Autodesk Inventor part; units mm, degrees
ref_plane "Work Plane1" through (29, 0, 0) normal (0, -1, 0) x (1, 0, 0)
ref_plane "YZ Plane" through (0, 0, 0) normal (1, 0, 0) x (0, 1, 0)
ref_plane "XZ Plane" through (0, 0, 0) normal (0, 1, 0) x (-1, 0, 0)
sketch "Skizze1" plane through (0, 0, 0) normal (0, 0, 1) x (1, 0, 0)
  line L0 (-2, 0) -> (50, 0)
  line L1 (50, 0) -> (50, 4)
  line L2 (50, 4) -> (22, 4)
  line L3 (22, 4) -> (21.2331, 4)
  line L4 (21.2331, 4) -> (0, 4)
  line L5 (0, 4) -> (0, 6.5)
  line L6 (0, 6.5) -> (-8, 6.5)
  line L7 (-8, 6.5) -> (-8, 3.4641)
  line L8 (-8, 3.4641) -> (-4, 3.4641)
  line L9 (-4, 3.4641) -> (-2, 0)
  line L10 (-19.6, 0) -> (61.6, 0)
  line L11 (0, -1.3) -> (0, 7.8)
  line L12 (22, 4) -> (0, 4) construction
  dimension "d1" = 28
  dimension "d2" = 0.7669
  dimension "d3" = 8
  dimension "d4" = 4
  dimension "d5" = 60
  dimension "d6" = 8
  dimension "d7" = 8
  dimension "d8" = 6.9282
  dimension "d9" = 13
  dimension "d26" = 50
revolve "Körper" add sketch "Skizze1" angle 360 about axis through (-2, 0, 0) along (1, 0, 0)
sketch "Skizze2" plane through (-8, 0, 0) normal (-1, 0, 0) x (0, 0, 1)
  circle A0 centre (0, 0) radius 3.4641
  line L0 (0, -9.1) -> (0, 9.1)
  line L1 (-9.1, 0) -> (9.1, 0)
  line L2 (3.4641, 0) -> (1.7321, -3)
  line L3 (1.7321, -3) -> (-1.7321, -3)
  line L4 (-1.7321, -3) -> (-3.4641, 0)
  line L5 (-3.4641, 0) -> (-1.7321, 3)
  line L6 (-1.7321, 3) -> (1.7321, 3)
  line L7 (1.7321, 3) -> (3.4641, 0)
extrude "Loch" add sketch "Skizze2" against normal up to next contours L7 A0 | A0 L2 | L6 L0 A0 | A0 L0 L3 | L0 L6 A0 | A0 L3 L0 | L4 A0 | A0 L5
fillet "Rundung1" radius 0.8 1 edges at (-8, -6.5, 0)
thread "Gewinde"
chamfer "Fase1" distance 0.7668 distance2 0.7668 1 edges at (50, -4, 0) measured on face at (50, -0.3588, -0.308)
ref_plane "Work Plane1" through (29, 0, 0) normal (0, -1, 0) x (1, 0, 0)
fillet "Fillet2" radius 0.4 1 edges at (0, -4, 0)
equation "\"d1\" = GEL"
equation "\"d3\" = KOH"
equation "\"d4\" = INTI"
equation "\"d6\" = GD"
equation "\"d7\" = BDM"
equation "\"d8\" = 1.1547 * SW"
equation "\"d9\" = KOD"
equation "\"d26\" = NLG"
equation "\"d30\" = R"
equation "\"d17\" = RR"
equation "\"d13\" = GEL"
equation "\"d15\" = -0.5 * SPD + 0.5 * GD"
equation "\"d16\" = GUL"
equation "\"GD\" = NND"
equation "\"NLG\" = 50"
equation "\"GEL\" = 28"
equation "\"KOD\" = 13"
equation "\"KOH\" = 8"
equation "\"INTI\" = 4"
equation "\"GAL\" = 0.61345 * PTC"
equation "\"GUL\" = 0.61345 * PTC"
equation "\"BDM\" = NND"
equation "\"SW\" = 6"
equation "\"RR\" = 0.8"
equation "\"SPD\" = NND - 1.2269 * PTC"
equation "\"R\" = 0.4"
equation "\"TOA\" = 30deg"
equation "\"GD1\" = THREADDIA - 1.2269 * PTC"
equation "\"THREADDIA\" = 8"
equation "\"FAWI\" = 45deg"
equation "\"ANG\" = 120deg"
equation "\"PTC\" = 1.25"
equation "\"NND\" = 8"
equation "\"E0\" = 1.155 * SW"
properties part number "DIN 912 - M8 x 50" material "Stahl, weich"
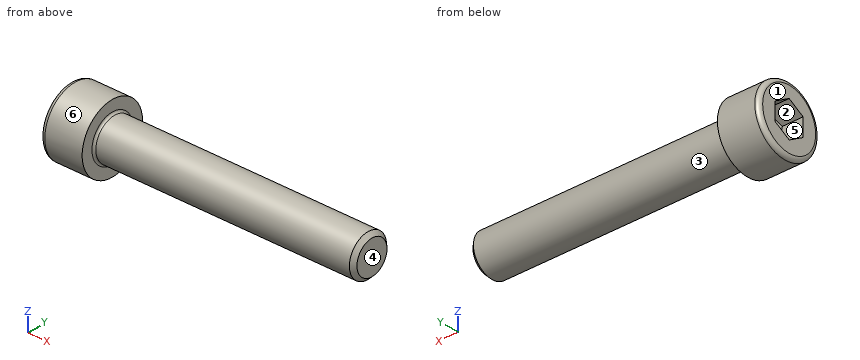
Can you work these out from the model? Positions are in its coordinate system, mm. Face numbers are marked on the shaded views. A direction names the side the tool comes from. Coordinates: 2 decimals unless noted, no trailing zeros. Write each loop counter-clockwise with the first axis right and the second up, starting at its lowest first coordinate (ties: lowest second). Pieces come first, ordered by that corner, then holes. Notation, with made-up numbers: (62.25, 1) - (84.25, 1) arc R7 cw to (84.25, 12) - close; hole circle Ø2 at (-34.5, 7). An arc over 180 degrees is marked (long way). Return JSON: item names as keys, results as strings. Group by question number.
Item 1: We'd pull the mould along Y, two halves only. Please class the marked faces 4, 5 and 6: pulls with the +Y half, pulls with the -Y half, needs draft (parallel to the pull), parting line crosses it, or undercut.
Item 2: If we section it at A-A (x = 23): Write out the boundary of the cut face in (y, z).
Item 3: Which directions (+Z, -Z, +X, -X, +Y, -Y) give clear straight access to the entire face, cutting with the end or side of a thin tool? Please do the marked faces 1, 2 and 3.
Item 4: Please list where these lines run through material, in increasing order: probe 1 along X at (y, z) = (5, 1.75); probe 2 along Z at (x, y) = (36.5, -2); probe 3 along Y at (x, z) = (18, 1.75).
Item 5: I'm going to push flat-ended pins straight in: pin 1 Ø2 at (x, y) = (4, -1) entering from +Z; pin 2 Ø3 at (x, z) = (32.5, 2) entering from +Y; pin 3 Ø4 at (x, y) = (14, 4) entering from -Z. Where does each tip first touch, or does it pass through?
Return value:
{
 "1": {"face 4": "needs draft", "face 5": "undercut", "face 6": "parting line crosses it"},
 "2": {"outline": "circle Ø8 at (0, 0)"},
 "3": {"face 1": "+Z, -Z, -X, +Y, -Y", "face 2": "-X", "face 3": "+X"},
 "4": {"probe 1": "x = -8 to 0", "probe 2": "z = -3.46 to 3.46", "probe 3": "y = -3.6 to 3.6"},
 "5": {"pin 1": "stops at z = 4", "pin 2": "stops at y = 3.97", "pin 3": "stops at z = -3.46"}
}
